```python
from build123d import *

# Parameters (mm, degrees)
F0_R     = 31.612422
F1_DEPTH = 71
F2_T     = -2.5
F3_R     = 10.164072
F4_DEPTH = 100


with BuildPart() as f1:
    # F0 (on Top) → F1 (new body)
    with BuildSketch(Plane.XY):
        Circle(F0_R)
    extrude(amount=F1_DEPTH)

    # F2
    f2_openings = [f1.faces().sort_by_distance(p)[0] for p in [
        (0, 0, 71),
    ]]
    offset(amount=F2_T, openings=f2_openings)

    # F3 (on Front) → F4 (cut)
    with BuildSketch(Plane.XZ):
        with Locations((2.623318, 32.751575)):
            Circle(F3_R)
    extrude(amount=-F4_DEPTH, mode=Mode.SUBTRACT)


solid = f1.part
```
Here's how the part is built. I have some questions about the finished solid (model axes, mm). A direction names the side the tool comes from. Round coordinates to 2 decimals unless told otherwise and drop trailing zeros. Loops run counter-clockwise (first coordinate to the right, second up) from the corner with the lowest first, then second, coordinate; pieces in that order, holes last. Notation, with made-up numbers: (-14, 46) -> (30, 46) arc R20 ccw to (30, 85) -> close; hole circle Ø4 at (80.5, 54.25). An arc over 180 degrees is marked (long way). Answer as CSV lines item,"result". Start each with the question number.
1. Imagine slicing it at D-D on z = 6. Write out the boundary of the cut face in (x, y), plus the area to 3 significant figures.
2. If we mould it in two halves opening along Y, with no side actions, what happens to faces 4 (the face through (-6.85, -30.86, 35)), 5 (the face through (14, -26, 71)), 6 (the face through (0, 0, 2.5))? For each: pulls with the +Y half, pulls with the -Y half, needs draft (parallel to the pull), parting line crosses it, or undercut.
3. For faces 1 (the face through (0, 0, 0)), 2 (the face through (-6.31, -28.42, 36.27)), 3 (the face through (7.313, 29.459, 23.734)), which set-ups out of +Z, -Z, +X, -X, +Y, -Y let a thin tool reach every point of the face, with its end or its side?
4. Imagine slicing it at B-B on x = 6.5. Write out the boundary of the cut face in (y, z).
5. I'm going to push flat-ended pins straight in: P1, Ø12, axis at y = 21.5, z = 59.5, coming from the +X side; P2, Ø1.5, axis at x = 17, y = -18, coming from the +Z side; P3, Ø5, axis at x = 6, z = 30, coming from the +Y side. Where does each tip first touch, or does it pass through?
6. I need wall thicknesses on probe 1 along Y at (x, z) = (0, 43.5); probe 2 along Z at (x, y) = (-25, -6); probe 3 along X at (y, z) = (-5, 40.5). Which ranges of each line are inside material? Lowest first, please. Write a range as from..to.
7. Imagine slicing it at C-C on x = 19. Write out the boundary of the cut face in (y, z), plus the area to 3 significant figures.
8. Imagine slicing it at A-A on y = 0. Write out the boundary of the cut face in (x, z), plus the area to 3 significant figures.
Solution:
1,outline,"circle Ø63.22 at (0, 0); hole circle Ø58.22 at (0, 0)"
1,area,"477 mm²"
2,face 4,"parting line crosses it"
2,face 5,"needs draft"
2,face 6,"undercut"
3,face 1,"-Z, +X, -X, +Y, -Y"
3,face 2,"+Z"
3,face 3,"+Y"
4,outline,"(-30.94, 0) -> (30.94, 0) -> (30.94, 23.36) -> (28.38, 23.36) -> (28.38, 2.5) -> (-28.38, 2.5) -> (-28.38, 71) -> (-30.94, 71) -> close; (28.38, 42.15) -> (30.94, 42.15) -> (30.94, 71) -> (28.38, 71) -> close"
5,P1,"x = 27.55"
5,P2,"z = 2.5"
5,P3,"y = -27.84"
6,probe 1,"-31.61..-29.11, 29.11..31.61"
6,probe 2,"0..2.5"
6,probe 3,"-31.21..-28.68, 28.68..31.21"
7,outline,"(-25.27, 0) -> (25.27, 0) -> (25.27, 71) -> (22.06, 71) -> (22.06, 2.5) -> (-22.06, 2.5) -> (-22.06, 71) -> (-25.27, 71) -> close"
7,area,"566 mm²"
8,outline,"(-31.61, 0) -> (31.61, 0) -> (31.61, 71) -> (29.11, 71) -> (29.11, 2.5) -> (-29.11, 2.5) -> (-29.11, 71) -> (-31.61, 71) -> close"
8,area,"501 mm²"
